from build123d import *

# Parameters (mm, degrees)
F0_W      = 127
F0_H      = 127
F1_DEPTH  = 101.6
F2_W      = 101.6
F2_H      = 88.9
F3_DEPTH  = 114.3
F4_R      = 15.875
F5_DEPTH  = 127.001
F6_R      = 5.08
F8_DEPTH  = 127
F9_W      = 137.247718
F9_H      = 152.4
F10_DEPTH = 127


with BuildPart() as f1:
    # F0 (on Top) → F1 (new body)
    with BuildSketch(Plane.XY):
        with Locations((63.5, 63.5)):
            Rectangle(F0_W, F0_H)
    extrude(amount=-F1_DEPTH)

    # F2 (on face) → F3 (cut)
    with BuildSketch(Plane.YZ.offset(127)):
        with Locations((63.5, -57.15)):
            Rectangle(F2_W, F2_H)
    extrude(amount=-F3_DEPTH, mode=Mode.SUBTRACT)

    # F4 (on face) → F5 (cut, through all)
    with BuildSketch(Plane.XZ):
        with Locations((101.6, -50.8)):
            Circle(F4_R)
    extrude(amount=-F5_DEPTH, mode=Mode.SUBTRACT)

    # F6
    f6_edges = [f1.edges().sort_by_distance(p)[0] for p in [
        (127, 63.5, 0),
    ]]
    fillet(f6_edges, radius=F6_R)

    # F7 (on face) → F8 (join)
    with BuildSketch(Plane.XZ):
        Polygon((0, -101.6), (0, 0), (-272.546083, -219.168201), (-135.084967, -219.168201), align=None)
    extrude(amount=-F8_DEPTH)

    # F9 (on face) → F10 (join)
    with BuildSketch(Plane.XZ):
        with Locations((-203.922224, -295.368201)):
            Rectangle(F9_W, F9_H)
    extrude(amount=-F10_DEPTH)


solid = f1.part
Could you check a few things on this model? Use its own coordinates, in mm. A direction names the side the tool comes from. Round coordinates to 2 decimals unless told otherwise and drop trailing zeros. Write each loop counter-clockwise with the first axis right and the second up, starting at its lowest first coordinate (ties: lowest second). Pieces come first, ordered by that corner, then holes. Notation, with made-up numbers: (76, -31) - (120, -31) arc R22 cw to (120, -25) - close; hole circle Ø2 at (73, 76). An arc over 180 degrees is marked (long way). Put each result on its own line as item: value. Start each with the question number.
(1) I want a section at B-B, the plane z = -50.8. Please give me the cut outline in (x, y) (3 decimals), plus the area to 3 significant figures.
(2) I need wall thicknesses on probe 1 along Z at (x, y) = (101.6, 5) (3 decimals); probe 2 along Z at (x, y) = (31, 64); probe 3 along X at (y, z) = (33, -331.5). Which ranges of each line are inside material? Lowest first, please.
(3) I want a section at D-D, the plane x = 41. Please give me the cut outline in (y, z), plus the area to 3 significant figures.
(4) Thinking about a two-plate mould opening in Y: for faces 4 (the flat face through (-120, 127, -183)), 5 (the flat face through (-120, 0, -183)), 6 (the flat face through (71, 12.7, -58)), 7 (the flat face through (71, 114.3, -58)), which applies, released by +Y, released by -Y, zero draft, split by the parting line, or undercut?
(5) Will these pins go through, and if not, where does the flat tip stop? pin 1 (10 mm diameter, centred on y = 95, z = -325.5, fed in from +X); pin 2 (5 mm diameter, centred on x = -209.5, y = 82.5, fed in from +Z); pin 3 (3 mm diameter, centred on y = 50, z = -176, fed in from +X); pin 4 (19 mm diameter, centred on x = 101.6, z = -50.8, fed in from -Y).
(6) For faces 1 (the flat face through (12.7, 63, -57)), 2 (the flat face through (11, 64, -101.6)), 3 (the flat face through (-272.546, 63, -296)), which set-ups out of +Z, -Z, +X, -X, +Y, -Y let a thin tool reach every point of the face, with its end or its side?
(7) I want a section at A-A, the plane x = 101.6. Please give me the cut outline in (y, z) (3 decimals).
(8) I want a section at C-C, the plane y = 24.5. Please give me the cut outline in (x, z).
Here are the results:
1. outline: (-63.172, 0) - (85.725, 0) - (85.725, 12.7) - (12.7, 12.7) - (12.7, 114.3) - (85.725, 114.3) - (85.725, 127) - (-63.172, 127) - close; (117.475, 0) - (127, 0) - (127, 12.7) - (117.475, 12.7) - close; (117.475, 114.3) - (127, 114.3) - (127, 127) - (117.475, 127) - close
1. area: 11,700 mm^2
2. probe 1: z = -101.6 to -66.675, -34.925 to 0
2. probe 2: z = -12.7 to 0
2. probe 3: x = -272.55 to -135.3
3. outline: (0, -101.6) - (12.7, -101.6) - (12.7, -12.7) - (114.3, -12.7) - (114.3, -101.6) - (127, -101.6) - (127, 0) - (0, 0) - close
3. area: 3,870 mm^2
4. face 4: released by +Y
4. face 5: released by -Y
4. face 6: undercut
4. face 7: undercut
5. pin 1: stops at x = -135.3
5. pin 2: stops at z = -166.46
5. pin 3: stops at x = -83.76
5. pin 4: passes through
6. face 1: -Z, +X
6. face 2: -Z, +X, +Y, -Y
6. face 3: +Z, -Z, -X, +Y, -Y
7. outline: (0, -101.6) - (12.7, -101.6) - (12.7, -66.675) - (0, -66.675) - close; (0, -34.925) - (12.7, -34.925) - (12.7, -12.7) - (114.3, -12.7) - (114.3, -34.925) - (127, -34.925) - (127, 0) - (0, 0) - close; (114.3, -101.6) - (127, -101.6) - (127, -66.675) - (114.3, -66.675) - close
8. outline: (-272.55, -371.57) - (-135.3, -371.57) - (-135.3, -219.17) - (-135.08, -219.17) - (0, -101.6) - (12.7, -101.6) - (12.7, -12.7) - (127, -12.7) - (127, -5.08) arc R5.08 ccw to (121.92, 0) - (0, 0) - (-272.55, -219.17) - close
